```python
from build123d import *

# Parameters (mm, degrees)
CROQUIS1_W              = 240
CROQUIS1_H              = 200
SALIENTE_EXTRUIR1_DEPTH = 3
CROQUIS2_W              = 3
CROQUIS2_H              = 29.2
CROQUIS2_W_2            = 24.85
CROQUIS2_H_2            = 3
CROQUIS2_W_3            = 49.7
CROQUIS2_W_4            = 66.784595416
CORTAR_EXTRUIR1_DEPTH   = 4
SALIENTE_EXTRUIR2_DEPTH = 3
REDONDEO1_R             = 1.5


with BuildPart() as part:
    # Croquis1 → Saliente-Extruir1 (new body)
    with BuildSketch(Plane.XY):
        Rectangle(CROQUIS1_W, CROQUIS1_H)
    extrude(amount=SALIENTE_EXTRUIR1_DEPTH)

    # Croquis2 → Cortar-Extruir1 (cut, through all)
    with BuildSketch(Plane(origin=(0, 0, 0), x_dir=(-1, 0, 0), z_dir=(0, 0, -1))):
        with Locations((-118.5, -66)):
            Rectangle(CROQUIS2_W, CROQUIS2_H)
        with Locations((-118.5, -21)):
            Rectangle(CROQUIS2_W, CROQUIS2_H)
        with Locations((-118.5, 24)):
            Rectangle(CROQUIS2_W, CROQUIS2_H)
        with Locations((-118.5, 69)):
            Rectangle(CROQUIS2_W, CROQUIS2_H)
        with Locations((107.575, -98.5)):
            Rectangle(CROQUIS2_W_2, CROQUIS2_H_2)
        with Locations((20, -98.5)):
            Rectangle(CROQUIS2_W_3, CROQUIS2_H_2)
        with Locations((-88.542297708, -98.5)):
            Rectangle(CROQUIS2_W_4, CROQUIS2_H_2)
        with Locations((118.5, -66)):
            Rectangle(CROQUIS2_W, CROQUIS2_H)
        with Locations((118.5, -21)):
            Rectangle(CROQUIS2_W, CROQUIS2_H)
        with Locations((118.5, 24)):
            Rectangle(CROQUIS2_W, CROQUIS2_H)
        with Locations((118.5, 69)):
            Rectangle(CROQUIS2_W, CROQUIS2_H)
    extrude(amount=-CORTAR_EXTRUIR1_DEPTH, mode=Mode.SUBTRACT)

    # Croquis3 → Saliente-Extruir2 (add)
    with BuildSketch(Plane(origin=(0, 0, 0), x_dir=(-1, 0, 0), z_dir=(0, 0, -1))):
        with BuildLine():
            Line((-55, 100), (-55, 104.8))
            ThreePointArc((-55, 104.8), (-54.560660172, 105.860660172), (-53.5, 106.3))
            Line((-53.5, 106.3), (-41.5, 106.3))
            ThreePointArc((-41.5, 106.3), (-40.439339828, 106.739339828), (-40, 107.8))
            Line((-40, 107.8), (-40, 112.8))
            ThreePointArc((-40, 112.8), (-40.439339828, 113.860660172), (-41.5, 114.3))
            Line((-41.5, 114.3), (-78.5, 114.3))
            ThreePointArc((-78.5, 114.3), (-79.560660172, 113.860660172), (-80, 112.8))
            Line((-80, 112.8), (-80, 100))
            Line((-80, 100), (-55, 100))
        make_face()
        with BuildLine():
            Line((0, 100), (25, 100))
            Line((25, 100), (25, 104.8))
            ThreePointArc((25, 104.8), (25.439339828, 105.860660172), (26.5, 106.3))
            Line((26.5, 106.3), (38.5, 106.3))
            ThreePointArc((38.5, 106.3), (39.560660172, 106.739339828), (40, 107.8))
            Line((40, 107.8), (40, 112.8))
            ThreePointArc((40, 112.8), (39.560660172, 113.860660172), (38.5, 114.3))
            Line((38.5, 114.3), (1.5, 114.3))
            ThreePointArc((1.5, 114.3), (0.439339828, 113.860660172), (0, 112.8))
            Line((0, 112.8), (0, 100))
        make_face()
    extrude(amount=-SALIENTE_EXTRUIR2_DEPTH)

    # Redondeo1
    redondeo1_edges = [part.edges().sort_by_distance(p)[0] for p in [
        (55, 100, 1.5),
        (80, 100, 1.5),
        (-25, 100, 1.5),
        (0, 100, 1.5),
    ]]
    fillet(redondeo1_edges, radius=REDONDEO1_R)


solid = part.part
```
Geometry: final body of the model. Coordinates: model frame, mm. Round coordinates to 2 decimals unless told otherwise and drop trailing zeros. Write each loop counter-clockwise with the first axis right and the second up, starting at its lowest first coordinate (ties: lowest second). Pieces come first, ordered by that corner, then holes. Notation, with made-up numbers: M 66.25,26.25 L 125.25,26.25 A15 ccw 125.25,47.25 Z; hole C -2,55 d10. An arc over 180 degrees is marked long. Answer in a Markdown table with one row per item. Add a question column.
(1) Cut plane B-B, the plane y = -19. Return the cut outline in (x, z), then the cut area to 3 significant figures.
(2) Contact query for flat-ended pins moving along their axis: pin 1 (0.9 mm diameter, centred on y = -60, z = 1.5, fed in from -X); pin 2 (1.5 mm diameter, centred on x = 119, z = 2, fed in from -Y); pin 3 (1 mm diameter, centred on y = -69.5, z = 2, fed in from +X). Output: stop coordinate, or through.
(3) Cut plane A-A, the plane x = 47. Return the cut outline in (y, z), then the cut area to 3 significant figures.
(4) Ray query, L1, parallel to Y at x = 47.5, z = 0.6; L2, parallel to X at y = 17, z = 0.6; L3, parallel to Y at x = 59, z = 1.35. Return the intervals inside material, ascending.
(5) Cut plane C-C, the plane x = -102.5. Return the cut outline in (y, z).
Established:
| question | item | result |
|---|---|---|
| 1 | outline | M -117,0 L 117,0 L 117,3 L -117,3 Z |
| 1 | area | 702 mm² |
| 2 | pin 1 | x = -117 |
| 2 | pin 2 | y = -97 |
| 2 | pin 3 | x = 117 |
| 3 | outline | M -100,0 L 100,0 L 100,3 L -100,3 Z; M 106.3,0 L 114.3,0 L 114.3,3 L 106.3,3 Z |
| 3 | area | 624 mm² |
| 4 | L1 | -100 to 100, 106.3 to 114.3 |
| 4 | L2 | -117 to 117 |
| 4 | L3 | -97 to 114.3 |
| 5 | outline | M -97,0 L 100,0 L 100,3 L -97,3 Z |
